Source: CAD feature listing. Evaluate the final solid. Frame: model axes, mm. A direction names the side the tool comes from. Round coordinates to 2 decimals unless told otherwise and drop trailing zeros. Order: outer loops, then holes, each group sorted by start corner. A loop starts at its lowest first (then second) coordinate and runs counter-clockwise, first axis right, second up. Notation, with made-up numbers: (48, 22.5) -> (96, 22.5) arc R10 cw to (96, 31.5) -> close; hole circle Ø3 at (46, -19). An arc over 180 degrees is marked (long way). Answer as CSV lines item,"result".
from build123d import *

# Parameters (mm, degrees)
BASE_FLANGE1_DEPTH     = 6
SKETCHED_START         = -80
SKETCHED_BEND1_DEPTH   = 38
SKETCHED_START_2       = 42
SKETCHED_BEND1_2_DEPTH = 38
SKETCHED_BEND1_3_DEPTH = 38
SKETCHED_BEND1_4_DEPTH = 38


# Read off the part's stored shape, not the designer's step: Sketched Bend1
# Sheet-metal steps are written as plain solids
with BuildPart() as part:
    # Sketch1 → Base-Flange1 (new body)
    with BuildSketch(Plane.XY):
        with BuildLine():
            Line((80, 189.59), (80, 54.12))
            ThreePointArc((80, 54.12), (79.87085305, 52.518044922), (79.486747986, 50.957467367))
            Line((79.486747986, 50.957467367), (42.276747986, -60.662532633))
            ThreePointArc((42.276747986, -60.662532633), (38.636993829, -65.612500426), (32.79, -67.5))
            Line((32.79, -67.5), (5, -67.5))
            Line((5, -67.5), (5, -52.5))
            ThreePointArc((5, -52.5), (0, -47.5), (-5, -52.5))
            Line((-5, -52.5), (-5, -67.5))
            Line((-5, -67.5), (-32.79, -67.5))
            ThreePointArc((-32.79, -67.5), (-38.636993829, -65.612500426), (-42.276747986, -60.662532633))
            Line((-42.276747986, -60.662532633), (-79.486747986, 50.957467367))
            ThreePointArc((-79.486747986, 50.957467367), (-79.87085305, 52.518044922), (-80, 54.12))
            Line((-80, 54.12), (-80, 189.59))
            Line((-80, 189.59), (-80, 249.59))
            Line((-80, 249.59), (-42, 249.59))
            Line((-42, 249.59), (-42, 189.59))
            Line((-42, 189.59), (-39, 189.59))
            Line((-39, 189.59), (-39, 296.5))
            Line((-39, 296.5), (39, 296.5))
            Line((39, 296.5), (39, 189.59))
            Line((39, 189.59), (42, 189.59))
            Line((42, 189.59), (42, 249.59))
            Line((42, 249.59), (80, 249.59))
            Line((80, 249.59), (80, 189.59))
        make_face()
        with BuildLine():
            Line((7.5, 25), (7.5, -25))
            ThreePointArc((7.5, -25), (0, -32.5), (-7.5, -25))
            Line((-7.5, -25), (-7.5, 25))
            ThreePointArc((-7.5, 25), (0, 32.5), (7.5, 25))
        make_face(mode=Mode.SUBTRACT)
    extrude(amount=-BASE_FLANGE1_DEPTH)

    # Sketched Bend1 outline → Sketched Bend1 (cut)
    with BuildSketch(Plane.YZ.offset(SKETCHED_START)):
        with BuildLine():
            Line((249.59, 0), (206.989995997, 0))
            ThreePointArc((206.989995997, 0), (201.42820323, -4.422205102), (194.5, -6))
            Line((194.5, -6), (249.59, -6))
            Line((249.59, -6), (249.59, 0))
        make_face()
    extrude(amount=SKETCHED_BEND1_DEPTH, mode=Mode.SUBTRACT)

    # Sketched Bend1 2 outline → Sketched Bend1 2 (cut)
    with BuildSketch(Plane.YZ.offset(SKETCHED_START_2)):
        with BuildLine():
            Line((249.59, 0), (206.989995997, 0))
            ThreePointArc((206.989995997, 0), (201.42820323, -4.422205102), (194.5, -6))
            Line((194.5, -6), (249.59, -6))
            Line((249.59, -6), (249.59, 0))
        make_face()
    extrude(amount=SKETCHED_BEND1_2_DEPTH, mode=Mode.SUBTRACT)

    # Sketched Bend1 3 outline → Sketched Bend1 3 (add)
    with BuildSketch(Plane.YZ.offset(SKETCHED_START)):
        with BuildLine():
            Line((210.5, 10), (210.5, 44.669647752))
            Line((210.5, 44.669647752), (204.5, 44.669647752))
            Line((204.5, 44.669647752), (204.5, 10))
            ThreePointArc((204.5, 10), (201.571067812, 2.928932188), (194.5, 0))
            Line((194.5, 0), (206.989995997, 0))
            ThreePointArc((206.989995997, 0), (209.597018513, 4.700940458), (210.5, 10))
        make_face()
    extrude(amount=SKETCHED_BEND1_3_DEPTH)

    # Sketched Bend1 4 outline → Sketched Bend1 4 (add)
    with BuildSketch(Plane.YZ.offset(SKETCHED_START_2)):
        with BuildLine():
            Line((210.5, 10), (210.5, 44.669647752))
            Line((210.5, 44.669647752), (204.5, 44.669647752))
            Line((204.5, 44.669647752), (204.5, 10))
            ThreePointArc((204.5, 10), (201.571067812, 2.928932188), (194.5, 0))
            Line((194.5, 0), (206.989995997, 0))
            ThreePointArc((206.989995997, 0), (209.597018513, 4.700940458), (210.5, 10))
        make_face()
    extrude(amount=SKETCHED_BEND1_4_DEPTH)


solid = part.part
1. Section query D-D on y = 265.5. Return loops of the section in (x, z), and give its area (3 significant figures).
Results below:
outline,"(-39, -6) -> (39, -6) -> (39, 0) -> (-39, 0) -> close"
area,"468 mm2"
2. Section query C-C on x = -63.5. Return loops of the section in (y, z).
Results below:
outline,"(3, -6) -> (194.5, -6) arc R16 ccw to (210.5, 10) -> (210.5, 44.67) -> (204.5, 44.67) -> (204.5, 10) arc R10 cw to (194.5, 0) -> (3, 0) -> close"
3. Line query: L1, parallel to Z at x = -40, y = -23; L2, parallel to Y at x = -58, z = 13.5; L3, parallel to Y at x = -72.5, z = 8.5. Output: solid intervals per line, ascending. Write a range as [from, to].
Results below:
L1,"[-6, 0]"
L2,"[204.5, 210.5]"
L3,"[204.39, 210.43]"
4. Section query A-A on z = 36.5. Return loops of the section in (x, y), and give its area (3 significant figures).
Results below:
outline,"(-80, 204.5) -> (-42, 204.5) -> (-42, 210.5) -> (-80, 210.5) -> close; (42, 204.5) -> (80, 204.5) -> (80, 210.5) -> (42, 210.5) -> close"
area,"456 mm2"
5. Reachability of faces 1 (the flat face through (61, 204.5, 28)), 2 (the cylindrical face through (-38.57, -65.66, -2.96)), 3 (the flat face through (-42, 205, 20)), 4 (the flat face through (1, 117, -6)), 5 (the cylindrical face through (-0.16, 32.5, -2.96)) from +Z, -Z, +X, -X, +Y, -Y: full face, straight path, thin tool, end or side. Return the list, or none.
Results below:
face 1,"+Z, +X, -X, -Y"
face 2,"+Z, -Z, -X, -Y"
face 3,"+Z, -Z, +Y"
face 4,"-Z, +X, -X, +Y, -Y"
face 5,"+Z, -Z"
6. Pin query (flat end, axial travel): pin 1 (0.9 mm diameter, centred on x = -41, z = -3.5, fed in from +Y); pin 2 (3 mm diameter, centred on x = 51.5, z = 33, fed in from -Y); pin 3 (5 mm diameter, centred on y = 230.5, z = -3, fed in from +X). Return the tip coordinate at first contact, or that it passes through.
Results below:
pin 1,"y = 189.59"
pin 2,"y = 204.5"
pin 3,"x = 39"
7. Section query B-B on x = 0. Return loops of the section in (y, z), and give its area (3 significant figures).
Results below:
outline,"(-47.5, -6) -> (-32.5, -6) -> (-32.5, 0) -> (-47.5, 0) -> close; (32.5, -6) -> (296.5, -6) -> (296.5, 0) -> (32.5, 0) -> close"
area,"1,670 mm2"
